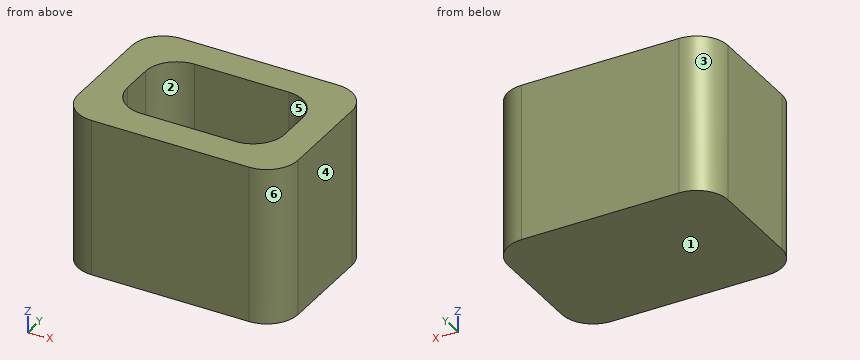
```python
from build123d import *

# Parameters (mm, degrees)
F0_W        = 177.8
F0_H        = 127
F1_DEPTH    = 127
F2_R        = 25.4
F3_T        = 25.4
F4_T1_DEPTH = 101.6


# Not quite as in the source:
# - a fillet or chamfer that OpenCascade refuses, or shapes differently, is made with other operations: its cross-section is extruded or revolved along the edge and cut away or added
# - a shell that OpenCascade refuses in one call is made with other operations: the cavity is built on its own and cut out


with BuildPart() as f1:
    # F0 (on Top) → F1 (new body)
    with BuildSketch(Plane.XY):
        with Locations((88.9, -63.5)):
            Rectangle(F0_W, F0_H)
    extrude(amount=F1_DEPTH)

    # F2
    f2_edges = [f1.edges().sort_by_distance(p)[0] for p in [
        (0, -127, 63.5),
        (177.8, -127, 63.5),
        (177.8, 0, 63.5),
        (0, 0, 63.5),
    ]]
    fillet(f2_edges, radius=F2_R)

    # F3: shell of thickness 25.4, made by hand


with BuildPart() as f3_core1:
    # F3_t2: copy of F1
    add(f1.part)

    # the walls: a layer under each face that stays
    f3_faces = [f3_core1.faces().sort_by_distance(p)[0] for p in [
        (88.9, 0, 63.5),
        (88.9, -63.5, 0),
        (177.8, -63.5, 63.5),
        (0, -63.5, 63.5),
        (88.9, -127, 63.5),
    ]]
    thicken(f3_faces, amount=-F3_T, mode=Mode.SUBTRACT)


with BuildPart() as f1_1:
    add(f1.part)

    # what is left inside the walls is the cavity
    f3_cavity = [f3_core1.part.solids().sort_by_distance(p)[0] for p in [
        (88.9, -25.654, 93.133333),
    ]]
    add(f3_cavity, mode=Mode.SUBTRACT)

    # F4: fillet of radius 25.4 on 6 edges, made by hand

    # F4_s2 → F4_t1 (join)
    with BuildSketch(Plane.XY.offset(25.4)):
        with BuildLine():
            ThreePointArc((50.8, -25.4), (32.8394877579, -32.8394877579), (25.4, -50.8))
            Line((25.4, -50.8), (25.4, -25.4))
            Line((25.4, -25.4), (50.8, -25.4))
        make_face()
        with BuildLine():
            ThreePointArc((127, -25.4), (144.9605122421, -32.8394877579), (152.4, -50.8))
            Line((152.4, -50.8), (152.4, -25.4))
            Line((152.4, -25.4), (127, -25.4))
        make_face()
        with BuildLine():
            ThreePointArc((25.4, -76.2), (32.8394877579, -94.1605122421), (50.8, -101.6))
            Line((50.8, -101.6), (25.4, -101.6))
            Line((25.4, -101.6), (25.4, -76.2))
        make_face()
        with BuildLine():
            ThreePointArc((127, -101.6), (144.9605122421, -94.1605122421), (152.4, -76.2))
            Line((152.4, -76.2), (152.4, -101.6))
            Line((152.4, -101.6), (127, -101.6))
        make_face()
    extrude(amount=F4_T1_DEPTH)


solid = f1_1.part
```
Source: CAD feature listing. Evaluate the final solid. Frame: model axes, mm. Face numbers are marked on the shaded views. A direction names the side the tool comes from. Coordinates: 2 decimals unless noted, no trailing zeros. Write each loop counter-clockwise with the first axis right and the second up, starting at its lowest first coordinate (ties: lowest second). Pieces come first, ordered by that corner, then holes. Notation, with made-up numbers: (-34, -24) -> (6, -24) arc R18 cw to (6, -13) -> close; hole circle Ø9 at (12.25, 56.5). An arc over 180 degrees is marked (long way). Return JSON: item names as keys, results as strings. Group by question number.
1) Ray query, line 1 along Y through (x, z) = (124.5, 76); line 2 along X through (y, z) = (-66.5, 85); line 3 along Z through (x, y) = (123, -53.5). Return the intervals inside material, ascending.
2) Contact query for a flat-ended pin moving along its axis: P1, Ø12, axis at x = 62.5, y = -54, coming from the -Z side. Output: stop coordinate, or through.
3) Mould query, pull axis X, two halves, no side actions, for the marked faces 1, 2, 3 and 4. Classes: +X half, -X half, draft (parallel to the pull), parting line (faces both ways), or undercut.
4) Section query A-A, the plane z = 31. Return loops of the section in (x, y), plus the area to 3 significant figures.
5) Section query C-C, the plane y = -70. Return loops of the section in (x, z).
6) Section query D-D, the plane y = -13.5. Return loops of the section in (x, z), plus the area to 3 significant figures.
7) Set-up query: the marked faces 5 and 6. Return all of +Z, -Z, +X, -X, +Y, -Y with unobstructed straight access to the full face (end or side cutting, diameter ignored); none if empty.
8) Section query B-B, the plane x = 98. Return loops of the section in (y, z), plus the area to 3 significant figures.
From the geometry:
{
 "1": {"line 1": "-127 to -101.6, -25.4 to 0", "line 2": "0 to 25.4, 152.4 to 177.8", "line 3": "0 to 25.4"},
 "2": {"P1": "z = 0"},
 "3": {"face 1": "draft", "face 2": "undercut", "face 3": "-X half", "face 4": "+X half"},
 "4": {"outline": "(0, -101.6) arc R25.4 ccw to (25.4, -127) -> (152.4, -127) arc R25.4 ccw to (177.8, -101.6) -> (177.8, -25.4) arc R25.4 ccw to (152.4, 0) -> (25.4, 0) arc R25.4 ccw to (0, -25.4) -> close; hole (25.4, -76.2) arc R25.4 ccw to (50.8, -101.6) -> (127, -101.6) arc R25.4 ccw to (152.4, -76.2) -> (152.4, -50.8) arc R25.4 ccw to (127, -25.4) -> (50.8, -25.4) arc R25.4 ccw to (25.4, -50.8) -> close", "area": "12,900 mm²"},
 "5": {"outline": "(0, 0) -> (177.8, 0) -> (177.8, 127) -> (152.4, 127) -> (152.4, 25.4) -> (25.4, 25.4) -> (25.4, 127) -> (0, 127) -> close"},
 "6": {"outline": "(2.96, 0) -> (174.84, 0) -> (174.84, 127) -> (2.96, 127) -> close", "area": "21,800 mm²"},
 "7": {"face 5": "+Z", "face 6": "+Z, -Z, +X, -Y"},
 "8": {"outline": "(-127, 0) -> (0, 0) -> (0, 127) -> (-25.4, 127) -> (-25.4, 25.4) -> (-101.6, 25.4) -> (-101.6, 127) -> (-127, 127) -> close", "area": "8,390 mm²"}
}
